from build123d import *

# Parameters (mm, degrees)
F0_W     = 20
F0_H     = 110
F1_DEPTH = 9
F3_DEPTH = 20
F4_T     = -2


with BuildPart() as f1:
    # F0 (on Top) → F1 (new body, symmetric)
    with BuildSketch(Plane.XY):
        with Locations((0, 5)):
            Rectangle(F0_W, F0_H)
    extrude(amount=F1_DEPTH, both=True)

    # F2 (on face) → F3 (cut)
    with BuildSketch(Plane.YZ.offset(10)):
        with BuildLine():
            ThreePointArc((-50, -9), (-49.2494239601, -197.6473192465), (114, -103.1063228481))
            ThreePointArc((114, -103.1063228481), (99.5409963984, -48.8568988881), (60, -9))
            Line((60, -9), (-50, -9))
        make_face()
        with BuildLine():
            Line((-50, -9), (60, -9))
            ThreePointArc((60, -9), (5, 5.8936771519), (-50, -9))
        make_face()
    extrude(amount=-F3_DEPTH, mode=Mode.SUBTRACT)

    # F4
    f4_openings = [f1.faces().sort_by_distance(p)[0] for p in [
        (10, -48.88537, 0),
    ]]
    offset(amount=F4_T, openings=f4_openings)


solid = f1.part
Could you check a few things on this model? Use its own coordinates, in mm. A direction names the side the tool comes from. Round coordinates to 2 decimals unless told otherwise and drop trailing zeros. Write each loop counter-clockwise with the first axis right and the second up, starting at its lowest first coordinate (ties: lowest second). Pieces come first, ordered by that corner, then holes. Notation, with made-up numbers: (39, 67) - (94, 67) arc R33 cw to (94, 102) - close; hole circle Ø5 at (25, 63). An arc over 180 degrees is marked (long way). Put each result on its own line as item: value. Start each with the question number.
(1) I want a section at A-A, the plane x = 1. Please give me the cut outline in (y, z).
(2) I want a section at D-D, the plane z = 4.75. Please give me the cut outline in (x, y).
(3) I want a section at B-B, the plane z = -2. Please give me the cut outline in (x, y), plus the area to 3 significant figures.
(4) For faces 1 (the flat face through (1, 58, 1)), 2 (the flat face through (10, -3, 6)), which set-ups out of +Z, -Z, +X, -X, +Y, -Y let a thin tool reach every point of the face, with its end or its side?
(5) Thinking about a two-plate mould opening in Z: for faces 3 (the cylindrical face through (0.14, 5.81, 5.89)), 4 (the flat face through (-10, 4.2, 6.1)), 5 (the cylindrical face through (1.13, 39.39, 2.43)), which applies, released by +Z, released by -Z, zero draft, split by the parting line, or undercut?
(6) Will these pins go through, and if not, where does the flat tip stop? pin 1 (1 mm diameter, centred on x = 6.5, y = -29.5, fed in from -Z); pin 2 (5.5 mm diameter, centred on x = -2, y = 44, fed in from -Z); pin 3 (4 mm diameter, centred on y = -24.5, z = -0.5, fed in from +X); pin 4 (5.5 mm diameter, centred on x = 1, y = -32.5, fed in from -Z).
(7) I need wall thicknesses on probe 1 along Y at (x, z) = (7.25, -4.25); probe 2 along Y at (x, z) = (2.75, -2.5); probe 3 along Z at (x, y) = (4.5, -38). Which ranges of each line are inside material? Lowest first, please.
(8) I want a section at C-C, the plane y = -36. Please give me the cut outline in (x, z).
Here are the results:
1. outline: (-50, -9) arc R109 cw to (60, -9) - (60, 9) - (-50, 9) - close; hole (-48, -5.58) arc R111 cw to (-9.06, 7) - (-48, 7) - close; hole (19.06, 7) arc R111 cw to (58, -5.58) - (58, 7) - close
2. outline: (-10, -50) - (10, -50) - (10, -48) - (-8, -48) - (-8, -21.23) - (10, -21.23) - (10, -10.75) - (-10, -10.75) - close; (-10, 20.75) - (10, 20.75) - (10, 31.23) - (-8, 31.23) - (-8, 58) - (10, 58) - (10, 60) - (-10, 60) - close
3. outline: (-10, -50) - (10, -50) - (10, -48) - (-8, -48) - (-8, -40.81) - (10, -40.81) - (10, -35.72) - (-10, -35.72) - close; (-10, 45.72) - (10, 45.72) - (10, 50.81) - (-8, 50.81) - (-8, 58) - (10, 58) - (10, 60) - (-10, 60) - close
3. area: 312 mm^2
4. face 1: +X
4. face 2: +Z, -Z, +X, +Y, -Y
5. face 3: released by -Z
5. face 4: zero draft
5. face 5: undercut
6. pin 1: stops at z = 0.12
6. pin 2: stops at z = -2.42
6. pin 3: passes through
6. pin 4: stops at z = -1.81
7. probe 1: y = -50 to -48, -45.48 to -40.92, 50.92 to 55.48, 58 to 60
7. probe 2: y = -50 to -48, -41.9 to -36.94, 46.94 to 51.9, 58 to 60
7. probe 3: z = -2.95 to -0.77, 7 to 9
8. outline: (-10, -2.11) - (10, -2.11) - (10, 0.04) - (-8, 0.04) - (-8, 7) - (10, 7) - (10, 9) - (-10, 9) - close
